Answer from the drawing. Dimensions are ordinates in mm from the lowest x, y and z of the part. A direction names the side the tool comes from. Round coordinates to 2 decimals unless told otherwise and drop trailing zeros. Write each loop counter-clockwise with the first axis right and the second up, starting at its lowest first coordinate (ties: lowest second). Pieces come first, ordered by that corner, then holes. Notation, with made-up numbers: (11, 64) -> (16, 64) arc R34 ccw to (16, 99) -> close; hole circle Ø8 at (-34, -4). An arc over 180 degrees is marked (long way). Return JSON: item names as keys, results as strings. Group by question number.
(1) A cutting plane is placed at C-C on y = 141.5. Give the vertices of the cut face in (x, z).
(2) Given pin 1 (4.5 mm diameter, centred on x = 167.5, y = 136.5, fed in from +Z); pin 2 (1 mm diameter, centred on x = 146.5, y = 90, fed in from -Z); pin 3 (12 mm diameter, centred on x = 118, y = 35.5, fed in from +Z), each flat-ended and moving along its own axis, determine where each tip first touches the part or whether it passes through.
(3) A cutting plane is placed at D-D on x = 35. Give the vertices of the cut face in (y, z), then the cut area to 3 significant figures.
(4) A cutting plane is placed at A-A on x = 100.5. Give the vertices of the cut face in (y, z).
(5) Straight lines are drawn through the part: line 1 (Y direction, x = 28, z = 141.5); line 2 (Y direction, x = 113.5, z = 123); line 3 (X direction, y = 137, z = 36). For each, find the intervals that lie inside material, in ascending order.
(6) For the marked faces 1, 2, 3, 4 and 5, determine the directions among +Z, -Z, +X, -X, +Y, -Y from which every point of the face is accessible in a straight line to the end or side of a thin tool.
(7) A cutting plane is placed at B-B on z = 100.5. Give the vertices of the cut face in (x, y), then the cut area to 3 significant figures.
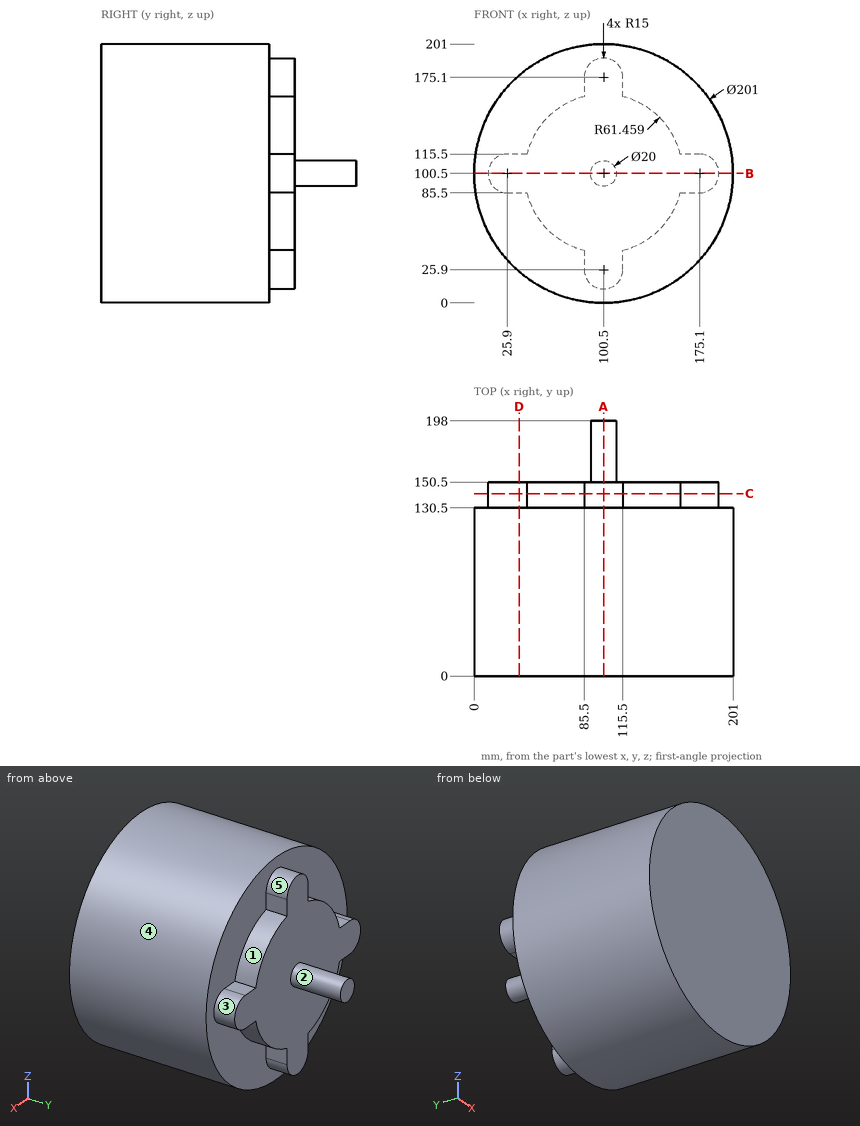
Checks:
{
 "1": {"outline": "(25.9, 85.5) -> (40.9, 85.5) arc R61.46 ccw to (85.5, 40.9) -> (85.5, 25.9) arc R15 ccw to (115.5, 25.9) -> (115.5, 40.9) arc R61.46 ccw to (160.1, 85.5) -> (175.1, 85.5) arc R15 ccw to (175.1, 115.5) -> (160.1, 115.5) arc R61.46 ccw to (115.5, 160.1) -> (115.5, 175.1) arc R15 ccw to (85.5, 175.1) -> (85.5, 160.1) arc R61.46 ccw to (40.9, 115.5) -> (25.9, 115.5) arc R15 ccw to start"},
 "2": {"pin 1": "stops at z = 115.5", "pin 2": "stops at z = 10.89", "pin 3": "stops at z = 200.34"},
 "3": {"outline": "(0, 24.28) -> (130.5, 24.28) -> (130.5, 85.5) -> (150.5, 85.5) -> (150.5, 115.5) -> (130.5, 115.5) -> (130.5, 176.72) -> (0, 176.72) -> close", "area": "20,500 mm^2"},
 "4": {"outline": "(0, 0) -> (130.5, 0) -> (130.5, 10.9) -> (150.5, 10.9) -> (150.5, 90.5) -> (198, 90.5) -> (198, 110.5) -> (150.5, 110.5) -> (150.5, 190.1) -> (130.5, 190.1) -> (130.5, 201) -> (0, 201) -> close"},
 "5": {"line 1": "y = 0 to 130.5", "line 2": "y = 0 to 150.5", "line 3": "x = 85.5 to 115.5"},
 "6": {"face 1": "+Z, +X, +Y", "face 2": "+Y", "face 3": "+X, +Y", "face 4": "+Y, -Y", "face 5": "+Z, +Y"},
 "7": {"outline": "(0, 0) -> (201, 0) -> (201, 130.5) -> (190.1, 130.5) -> (190.1, 150.5) -> (110.5, 150.5) -> (110.5, 198) -> (90.5, 198) -> (90.5, 150.5) -> (10.9, 150.5) -> (10.9, 130.5) -> (0, 130.5) -> close", "area": "30,800 mm^2"}
}
